```python
from build123d import *

# Parameters (mm, degrees)
LID_PLATE_DEPTH     = 2.4
DRIP_SKIRT_DEPTH    = 3.01
SKETCH3_W           = 25.3
SKETCH3_H           = 1.9
FRONT_SKIRT_L_DEPTH = 5.4
SKETCH4_W           = 25.3
SKETCH4_H           = 1.9
FRONT_SKIRT_R_DEPTH = 5.4
SKETCH5_R           = 1.7
SCREW_HOLES_DEPTH   = 4.4


with BuildPart() as part:
    # Sketch1 → Lid Plate (new body)
    with BuildSketch(Plane(origin=(0, 28, 0), x_dir=(1, 0, 0), z_dir=(0, 1, 0))):
        Polygon((-65.187005769, -126.3), (65.187005769, -126.3), (74.3, -117.187005769), (74.3, -11.9), (-74.3, -11.9), (-74.3, -117.187005769), align=None)
    extrude(amount=LID_PLATE_DEPTH)

    # Sketch2 → Drip Skirt (add)
    with BuildSketch(Plane(origin=(0, 25, 0), x_dir=(1, 0, 0), z_dir=(0, 1, 0))):
        Polygon((74.3, -11.9), (74.3, -117.187005769), (65.187005769, -126.3), (-65.187005769, -126.3), (-74.3, -117.187005769), (-74.3, -11.9), (-72.7, -11.9), (-72.7, -116.524264069), (-64.524264069, -124.7), (64.524264069, -124.7), (72.7, -116.524264069), (72.7, -11.9), align=None)
    extrude(amount=DRIP_SKIRT_DEPTH)

    # Sketch3 → Front Skirt L (add)
    with BuildSketch(Plane(origin=(0, 25, 0), x_dir=(1, 0, 0), z_dir=(0, 1, 0))):
        with Locations((-61.65, -10.95)):
            Rectangle(SKETCH3_W, SKETCH3_H)
    extrude(amount=FRONT_SKIRT_L_DEPTH)

    # Sketch4 → Front Skirt R (add)
    with BuildSketch(Plane(origin=(0, 25, 0), x_dir=(1, 0, 0), z_dir=(0, 1, 0))):
        with Locations((61.65, -10.95)):
            Rectangle(SKETCH4_W, SKETCH4_H)
    extrude(amount=FRONT_SKIRT_R_DEPTH)

    # Sketch5 → Screw Holes (cut)
    with BuildSketch(Plane(origin=(0, 27, 0), x_dir=(1, 0, 0), z_dir=(0, 1, 0))):
        with Locations(Location((-66.5, -18.5, 0), (0, 0, 270))):
            Circle(SKETCH5_R)
        with Locations(Location((66.5, -18.5, 0), (0, 0, 270))):
            Circle(SKETCH5_R)
        with Locations(Location((-64, -116, 0), (0, 0, 270))):
            Circle(SKETCH5_R)
        with Locations(Location((64, -116, 0), (0, 0, 270))):
            Circle(SKETCH5_R)
        with Locations(Location((-44, -24, 0), (0, 0, 270))):
            Circle(SKETCH5_R)
        with Locations(Location((-44, -98, 0), (0, 0, 270))):
            Circle(SKETCH5_R)
        with Locations(Location((44, -24, 0), (0, 0, 270))):
            Circle(SKETCH5_R)
        with Locations(Location((44, -98, 0), (0, 0, 270))):
            Circle(SKETCH5_R)
    extrude(amount=SCREW_HOLES_DEPTH, mode=Mode.SUBTRACT)


solid = part.part
```
Geometry: final body of the model. Coordinates: model frame, mm. A direction names the side the tool comes from. Round coordinates to 2 decimals unless told otherwise and drop trailing zeros. Write each loop counter-clockwise with the first axis right and the second up, starting at its lowest first coordinate (ties: lowest second). Pieces come first, ordered by that corner, then holes. Notation, with made-up numbers: (81, 35) -> (118, 35) arc R25 cw to (118, 64) -> close; hole circle Ø4 at (2.25, 61). An arc over 180 degrees is marked (long way). Use CSV: the item, a comma, the result in double quotes. Start each with the question number.
Q1. Section D-D (x = 15.5). Return loops of the section in (y, z), plus the area to 3 significant figures.
Q2. Section A-A (x = 44). Return loops of the section in (y, z).
Q3. Section B-B (z = 24). Return loops of the section in (x, y), plus the area to 3 significant figures.
Q4. Pull-direction query (Z, two-part tool) for faces 1 (the face through (-62, 28, 10)), 2 (the face through (-68, 29.2, 19.3)), 3 (the face through (-1, 30.4, 67)), 4 (the face through (42.5, 29.2, 24.8)); classes: pulls with the +Z half, pulls with the -Z half, needs draft (parallel to the pull), parting line crosses it, or undercut.
Q5. First-contact query: pin 1 Ø4 at (x, z) = (64, 116) entering from -Y; pin 2 Ø2.5 at (x, y) = (-23, 29.5) entering from -Z. Flat tips, straight axial feed; report the tip coordinate or a pass-through.
Q6. Section C-C (y = 27.15). Return loops of the section in (x, z), plus the area to 3 significant figures.
Q7. Line query: L1, parallel to X at y = 29.5, z = 98; L2, parallel to Z at x = 44, y = 29.05; L3, parallel to X at y = 29.4, z = 18.5. Output: solid intervals per line, ascending.
Q8. Reachability of faces 5 (the face through (69.807, 27.662, 121.68)), 6 (the face through (-1, 26, 124.7)) from +Z, -Z, +X, -X, +Y, -Y: full face, straight path, thin tool, end or side. Return the list, or none.
Result sheet:
1,outline,"(25, 124.7) -> (28, 124.7) -> (28, 11.9) -> (30.4, 11.9) -> (30.4, 126.3) -> (25, 126.3) -> close"
1,area,"279 mm²"
2,outline,"(25, 124.7) -> (28, 124.7) -> (28, 99.7) -> (30.4, 99.7) -> (30.4, 126.3) -> (25, 126.3) -> close; (28, 11.9) -> (30.4, 11.9) -> (30.4, 22.3) -> (28, 22.3) -> close; (28, 25.7) -> (30.4, 25.7) -> (30.4, 96.3) -> (28, 96.3) -> close"
3,outline,"(-74.3, 25) -> (-72.7, 25) -> (-72.7, 28) -> (-45.7, 28) -> (-45.7, 30.4) -> (-74.3, 30.4) -> close; (-42.3, 28) -> (42.3, 28) -> (42.3, 30.4) -> (-42.3, 30.4) -> close; (45.7, 28) -> (72.7, 28) -> (72.7, 25) -> (74.3, 25) -> (74.3, 30.4) -> (45.7, 30.4) -> close"
3,area,"350 mm²"
4,face 1,"pulls with the -Z half"
4,face 2,"undercut"
4,face 3,"needs draft"
4,face 4,"undercut"
5,pin 1,"y = 28"
5,pin 2,"z = 11.9"
6,outline,"(-74.3, 10) -> (-49, 10) -> (-49, 11.9) -> (-72.7, 11.9) -> (-72.7, 116.52) -> (-64.52, 124.7) -> (64.52, 124.7) -> (72.7, 116.52) -> (72.7, 11.9) -> (49, 11.9) -> (49, 10) -> (74.3, 10) -> (74.3, 117.19) -> (65.19, 126.3) -> (-65.19, 126.3) -> (-74.3, 117.19) -> close"
6,area,"679 mm²"
7,L1,"-74.3 to -45.7, -42.3 to 42.3, 45.7 to 74.3"
7,L2,"11.9 to 22.3, 25.7 to 96.3, 99.7 to 126.3"
7,L3,"-74.3 to -68.2, -64.8 to 64.8, 68.2 to 74.3"
8,face 5,"+Z, +X, +Y, -Y"
8,face 6,"-Y"
